```python
from build123d import *

# Parameters (mm, degrees)
PAD_DEPTH       = 40
PAD001_DEPTH    = 15
POCKET_DEPTH    = 20.151
SKETCH003_R     = 4.05
POCKET001_DEPTH = 14
CHAMFER_SIZE    = 2
CHAMFER001_SIZE = 2
CHAMFER002_SIZE = 1


with BuildPart() as part:
    # Sketch → Pad (new body, symmetric)
    with BuildSketch(Plane.XY):
        with BuildLine():
            Line((-11, 45), (-11, 0))
            ThreePointArc((-11, 0), (0, -11), (11, 0))
            ThreePointArc((11, 0), (8.5, 2.5), (6, 0))
            ThreePointArc((-6, 0), (0, -6), (6, 0))
            Line((-6, 0), (-6, 45))
            ThreePointArc((-6, 45), (-8.5, 47.5), (-11, 45))
        make_face()
    extrude(amount=PAD_DEPTH, both=True)

    # Sketch001 → Pad001 (join)
    with BuildSketch(Plane.XZ):
        with BuildLine():
            ThreePointArc((-11, 15.15), (-26.15, 0), (-11, -15.15))
            Line((-11, 15.15), (-11, -15.15))
        make_face()
    extrude(amount=-PAD001_DEPTH)

    # Sketch002 (on Face1 of Pad001) → Pocket (cut, through all)
    with BuildSketch(Plane.YZ.offset(-6)):
        with BuildLine():
            Line((108.94, 32), (47, 32))
            ThreePointArc((47, 32), (15, 0), (47, -32))
            Line((47, -32), (108.94, -32))
            Line((108.94, -32), (108.94, 32))
        make_face()
    extrude(amount=-POCKET_DEPTH, mode=Mode.SUBTRACT)

    # Sketch003 (on DatumPlane) → Pocket001 (cut)
    with BuildSketch(Plane(origin=(-3.316026, 0, 0), x_dir=(0.992546, 0.121869, 0), z_dir=(-0.121869, 0.992546, 0))):
        with Locations((-13.070263, 0)):
            Circle(SKETCH003_R)
    extrude(amount=POCKET001_DEPTH, mode=Mode.SUBTRACT)

    # Chamfer
    chamfer_edges = [part.edges().sort_by_distance(p)[0] for p in [
        (-21.712668, 15, -10.712668),
    ]]
    chamfer(chamfer_edges, length=CHAMFER_SIZE)

    # Chamfer001
    chamfer001_edges = [part.edges().sort_by_distance(p)[0] for p in [
        (-26.15, 0, 0),
    ]]
    chamfer(chamfer001_edges, length=CHAMFER001_SIZE)

    # Chamfer002
    chamfer002_edges = [part.edges().sort_by_distance(p)[0] for p in [
        (-20.564859, 0, 0),
    ]]
    chamfer(chamfer002_edges, length=CHAMFER002_SIZE)


solid = part.part
```
Read the model definition and answer for the solid it produces. Units are mm, in the model's axes. A direction names the side the tool comes from. Give positions to 0.01 mm unless a question says otherwise; leave off trailing zeros. Order: outer loops, then holes, each group sorted by start corner. A loop starts at its lowest first (then second) coordinate and runs counter-clockwise, first axis right, second up. Notation, with made-up numbers: (77.25, -28.75) -> (95.25, -28.75) arc R17 ccw to (95.25, -12.75) -> close; hole circle Ø1 at (62, 1.5). An arc over 180 degrees is marked (long way). Write item = value, one per line.
1. Straight lines are drawn through the part: line 1 along Y through (x, z) = (-12.5, 4.5); line 2 along X through (y, z) = (3.5, -21); line 3 along X through (y, z) = (-5.5, -5.5). For each, find the intervals that lie inside material, in ascending order.
Numbers:
line_1 = 0 to 15
line_2 = -11 to -6
line_3 = -9.53 to -2.4, 2.4 to 9.53
2. A cutting plane is placed at C-C, the plane z = 33.5. Write down the section's boundary in (x, y), and give its area (3 significant figures).
Numbers:
outline = (-11, 0) arc R11 ccw to (11, 0) arc R2.5 ccw to (6, 0) arc R6 cw to (-6, 0) -> (-6, 45) arc R2.5 ccw to (-11, 45) -> close
area = 378 mm²
3. Given pin 1 (4 mm diameter, centred on y = 18.5, z = 30.5, fed in from -X); pin 2 (12 mm diameter, centred on y = 15.5, z = -16.5, fed in from -X); pin 3 (10 mm diameter, centred on x = 4.5, z = 20, fed in from +Y), each flat-ended and moving along its own axis, determine where each tip first touches the part or whether it passes through.
Numbers:
pin_1 = -11
pin_2 = -21.37
pin_3 = 2.5
4. A cutting plane is placed at D-D, the plane y = 29. Write down the section's boundary in (x, z).
Numbers:
outline = (-11, -40) -> (-6, -40) -> (-6, -26.46) -> (-11, -26.46) -> close; (-11, 26.46) -> (-6, 26.46) -> (-6, 40) -> (-11, 40) -> close
5. The mould has two halves that part along Y. Classify faces 1 (the face through (-18.051, 12.296, -0.057)), 2 (the face through (-26.146, 7.423, 0.333)), 3 (the face through (0, -6, 1)): +Y half, -Y half, draft (parallel to the pull), parting line (faces both ways), or undercut.
Numbers:
face_1 = undercut
face_2 = draft
face_3 = +Y half
6. For faces 4 (the face through (-21, 0, 3)), 5 (the face through (-16, 15, 0)), 6 (the face through (-6, 12, 1)), determine the directions among +Z, -Z, +X, -X, +Y, -Y from which every point of the face is accessible in a straight line to the end or side of a thin tool.
Numbers:
face_4 = +Z, -Z, -X, -Y
face_5 = +Z, -Z, -X, +Y
face_6 = +Z, -Z, +Y
7. A cutting plane is placed at A-A, the plane y = -5. Write down the section's boundary in (x, z), and give its area (3 significant figures).
Numbers:
outline = (-9.8, -40) -> (-3.32, -40) -> (-3.32, 40) -> (-9.8, 40) -> close; (3.32, -40) -> (9.8, -40) -> (9.8, 40) -> (3.32, 40) -> close
area = 1,040 mm²
8. A cutting plane is placed at B-B, the plane y = 14. Write down the section's boundary in (x, z), and give its area (3 significant figures).
Numbers:
outline = (-11, -40) -> (-6, -40) -> (-6, 40) -> (-11, 40) -> (-11, 14.15) arc R14.15 ccw to (-11, -14.15) -> close
area = 715 mm²
